Check sheet for the modelled part. Datum: model origin and axes. Units: mm. A direction names the side the tool comes from. Give positions to 0.01 mm unless a question says otherwise; leave off trailing zeros. Write each loop counter-clockwise with the first axis right and the second up, starting at its lowest first coordinate (ties: lowest second). Pieces come first, ordered by that corner, then holes.
from build123d import *

# Parameters (mm, degrees)
F1_DEPTH = 76.2
F2_SIZE  = 25.4
F3_R     = 9.525
F4_DEPTH = 19.051
F5_W     = 38.1
F5_H     = 50.8
F6_DEPTH = 19.051


with BuildPart() as f1:
    # F0 (on Top) → F1 (new body)
    with BuildSketch(Plane.XY):
        Polygon((-70.440705, 25.967644), (-84.387472, 25.967644), (-84.387472, -37.532356), (29.912528, -37.532356), (29.912528, -18.482356), (-70.440705, -18.482356), align=None)
    extrude(amount=F1_DEPTH)

    # F2
    f2_edges = [f1.edges().sort_by_distance(p)[0] for p in [
        (-77.414089, 25.967644, 76.2),
    ]]
    chamfer(f2_edges, length=F2_SIZE)

    # F3 (on face) → F4 (cut, through all)
    with BuildSketch(Plane(origin=(0, -18.482356, 0), x_dir=(-1, 0, 0), z_dir=(0, 1, 0))):
        with Locations((37.905472, 38.1)):
            Circle(F3_R)
    extrude(amount=-F4_DEPTH, mode=Mode.SUBTRACT)

    # F5 (on face) → F6 (cut, through all)
    with BuildSketch(Plane(origin=(0, -18.482356, 0), x_dir=(-1, 0, 0), z_dir=(0, 1, 0))):
        with Locations((-10.862528, 38.1)):
            Rectangle(F5_W, F5_H)
    extrude(amount=-F6_DEPTH, mode=Mode.SUBTRACT)


solid = f1.part
1) Sectioned sample at B-B on y = -24. Record the boundary of the cut face in (x, z) (3 decimals), then the cut area to 3 significant figures.
2) Sectioned sample at D-D on z = 5.5. Record the boundary of the cut face in (x, y), then the cut area to 3 significant figures.
3) Sectioned sample at A-A on x = 1. Record the boundary of the cut face in (y, z).
4) Draft check along X on faces 1 (the flat face through (-84.387, -5, 38)), 2 (the flat face through (-28, -27, 76.2)), 3 (the flat face through (-8.187, -28, 38)), 4 (the cylindrical face through (-30.89, -27.87, 44.54)). Enter one of: +X half, -X half, draft (parallel to the pull), parting line (faces both ways), or undercut.
5) Access from +Z, -Z, +X, -X, +Y, -Y to the whole of each face (thin tool, end or side, straight path). Record for faces 5 (the flat face through (-41, -19, 0)), 6 (the flat face through (-31, -18.482, 29)), 7 (the flat face through (11, -28, 63.5)).
6) Gauge pin test, flat ends, axial feed: pin 1 (9.5 mm diameter, centred on y = -31.5, z = 27.5, fed in from +X); pin 2 (21 mm diameter, centred on x = 2.5, y = -30.5, fed in from -Z); pin 3 (4 mm diameter, centred on x = -35.5, z = 8.5, fed in from +Y); pin 4 (6 mm diameter, centred on y = 1, z = 36, fed in from +X). Record the tip position at first contact, or that the pin passes through.
7) Scan lines: L1, parallel to Z at x = 11, y = -21.5; L2, parallel to X at y = -30, z = 38; L3, parallel to X at y = -5.5, z = 10. Record each from-to range of solid material in increasing order.
8) Sectioned sample at C-C on z = 38.1. Record the boundary of the cut face in (x, y).
Answers below:
1. outline: (-84.387, 0) - (29.913, 0) - (29.913, 12.7) - (-8.187, 12.7) - (-8.187, 63.5) - (29.913, 63.5) - (29.913, 76.2) - (-84.387, 76.2) - close; hole circle Ø19.05 at (-37.905, 38.1)
1. area: 6,490 mm2
2. outline: (-84.39, -37.53) - (29.91, -37.53) - (29.91, -18.48) - (-70.44, -18.48) - (-70.44, 25.97) - (-84.39, 25.97) - close
2. area: 2,800 mm2
3. outline: (-37.53, 0) - (-18.48, 0) - (-18.48, 12.7) - (-37.53, 12.7) - close; (-37.53, 63.5) - (-18.48, 63.5) - (-18.48, 76.2) - (-37.53, 76.2) - close
4. face 1: -X half
4. face 2: draft
4. face 3: +X half
4. face 4: undercut
5. face 5: -Z, +X, -X, +Y, -Y
5. face 6: +Z, -Z, +X, +Y
5. face 7: +X, +Y, -Y
6. pin 1: stops at x = -8.19
6. pin 2: stops at z = 0
6. pin 3: stops at y = -18.48
6. pin 4: stops at x = -70.44
7. L1: z = 0 to 12.7, 63.5 to 76.2
7. L2: x = -84.39 to -47.43, -28.38 to -8.19
7. L3: x = -84.39 to -70.44
8. outline: (-84.39, -37.53) - (-47.43, -37.53) - (-47.43, -18.48) - (-70.44, -18.48) - (-70.44, 25.97) - (-84.39, 25.97) - close; (-28.38, -37.53) - (-8.19, -37.53) - (-8.19, -18.48) - (-28.38, -18.48) - close
